from build123d import *

# Parameters (mm, degrees)
SKETCH1_W           = 44.45
SKETCH1_H           = 50.8
BOSS_EXTRUDE1_DEPTH = 76.2
CUT_EXTRUDE1_REACH  = 93.801
SKETCH2_R           = 6.731
SKETCH3_R           = 9.906
CUT_EXTRUDE2_DEPTH  = 38.608
CUT_EXTRUDE3_DEPTH  = 6.35


with BuildPart() as part:
    # Sketch1 → Boss-Extrude1 (new, symmetric)
    with BuildSketch(Plane.XY):
        Rectangle(SKETCH1_W, SKETCH1_H)
    extrude(amount=BOSS_EXTRUDE1_DEPTH, both=True)

    # Sketch2 → Cut-Extrude1 (cut, up to next)
    with BuildSketch(Plane(origin=(22.225, 0, 0), x_dir=(0, 0, -1), z_dir=(1, 0, 0)), mode=Mode.PRIVATE) as cut_extrude1_sk1:
        with Locations((-49.2125, -1.524)):
            Circle(SKETCH2_R)
    cut_extrude1_tool1 = extrude(cut_extrude1_sk1.sketch, amount=-CUT_EXTRUDE1_REACH, mode=Mode.PRIVATE) & part.part
    # Sketch2 → Cut-Extrude1 (cut, up to next)
    with BuildSketch(Plane(origin=(22.225, 0, 0), x_dir=(0, 0, -1), z_dir=(1, 0, 0)), mode=Mode.PRIVATE) as cut_extrude1_sk2:
        with Locations((49.2125, -1.524)):
            Circle(SKETCH2_R)
    cut_extrude1_tool2 = extrude(cut_extrude1_sk2.sketch, amount=-CUT_EXTRUDE1_REACH, mode=Mode.PRIVATE) & part.part
    add(cut_extrude1_tool1.solids().sort_by_distance((22.225, -1.524, 49.2125))[0], mode=Mode.SUBTRACT)
    add(cut_extrude1_tool2.solids().sort_by_distance((22.225, -1.524, -49.2125))[0], mode=Mode.SUBTRACT)

    # Sketch3 → Cut-Extrude2 (cut)
    with BuildSketch(Plane(origin=(22.225, 0, 0), x_dir=(0, 0, -1), z_dir=(1, 0, 0))):
        with Locations((-49.2125, -1.524)):
            Circle(SKETCH3_R)
        with Locations((49.2125, -1.524)):
            Circle(SKETCH3_R)
    extrude(amount=-CUT_EXTRUDE2_DEPTH, mode=Mode.SUBTRACT)

    # Sketch4 → Cut-Extrude3 (cut)
    with BuildSketch(Plane.XZ.offset(25.4)):
        with BuildLine():
            Line((22.225, -12.890241244), (22.225, 21.531765175))
            Line((22.225, 21.531765175), (0.947246364, 18.89010908))
            ThreePointArc((0.947246364, 18.89010908), (-11.925153457, 4.320761965), (0.947246364, -10.248585149))
            Line((0.947246364, -10.248585149), (22.225, -12.890241244))
        make_face()
    extrude(amount=-CUT_EXTRUDE3_DEPTH, mode=Mode.SUBTRACT)


solid = part.part
Can you work these out from the model? Positions are in its coordinate system, mm. A direction names the side the tool comes from. Coordinates: 2 decimals unless noted, no trailing zeros. Write each loop counter-clockwise with the first axis right and the second up, starting at its lowest first coordinate (ties: lowest second). Pieces come first, ordered by that corner, then holes.
Q1. Imagine slicing it at A-A, the plane y = -22. List the corners of the cut face in (x, z) for me (3 decimals).
Results found:
outline: (-22.225, -76.2) - (22.225, -76.2) - (22.225, -12.89) - (0.947, -10.249) arc R14.681 cw to (0.947, 18.89) - (22.225, 21.532) - (22.225, 76.2) - (-22.225, 76.2) - close
Q2. For P1, Ø10, axis at x = 8, z = 1, coming from the -Y side; P2, Ø6, axis at y = -0.5, z = 44.5, coming from the +X side; P3, Ø12, axis at x = 5.5, z = -5.5, coming from the -Y side, each with a flat end and sliding along its axis, tell me the tip position at first contact or that it passes through.
Results found:
P1: stops at y = -19.05
P2: stops at x = -16.38
P3: stops at y = -25.4
Q3. Which directions (+Z, -Z, +X, -X, +Y, -Y) give clear straight access to the entire face, cutting with the end or side of a thin tool? Please do faces 5 (the face through (-19.263, -4.102, 42.995)), 6 (the face through (-16.383, -4, -56)), 7 (the face through (-11.922, -22.269, 4.618)).
Results found:
face 5: +X, -X
face 6: +X
face 7: +X, -Y
Q4. Imagine slicing it at C-C, the plane z = 44.5. List the corners of the cut face in (x, y) for me (3 decimals).
Results found:
outline: (-22.225, -25.4) - (22.225, -25.4) - (22.225, -10.237) - (-16.383, -10.237) - (-16.383, -6.33) - (-22.225, -6.33) - close; (-22.225, 3.282) - (-16.383, 3.282) - (-16.383, 7.189) - (22.225, 7.189) - (22.225, 25.4) - (-22.225, 25.4) - close
Q5. If we mould it in two halves opening along Z, with no side actions, what happens to faces 1 (the face through (0, 0, 76.2)), 2 (the face through (11.74, -22.27, 20.23)), 3 (the face through (0, 0, -76.2)), 4 (the face through (0, 25.4, 1))? For each: +Z half, -Z half, draft (parallel to the pull), parting line (faces both ways), or undercut.
Results found:
face 1: +Z half
face 2: undercut
face 3: -Z half
face 4: draft
Q6. Imagine slicing it at D-D, the plane y = -5. List the corners of the cut face in (x, z) for me (1 decimal), plus the area to 3 significant figures.
Results found:
outline: (-22.2, -76.2) - (22.2, -76.2) - (22.2, -58.5) - (-16.4, -58.5) - (-16.4, -55) - (-22.2, -55) - close; (-22.2, -43.4) - (-16.4, -43.4) - (-16.4, -39.9) - (22.2, -39.9) - (22.2, 39.9) - (-16.4, 39.9) - (-16.4, 43.4) - (-22.2, 43.4) - close; (-22.2, 55) - (-16.4, 55) - (-16.4, 58.5) - (22.2, 58.5) - (22.2, 76.2) - (-22.2, 76.2) - close
area: 5,210 mm2
Q7. Please list where these lines run through material, in increasing order: L1, parallel to Z at x = 9, y = -7; L2, parallel to Z at x = -10, y = -6; L3, parallel to Y at x = -7, z = -45.5.
Results found:
L1: z = -76.2 to -57.47, -40.96 to 40.96, 57.47 to 76.2
L2: z = -76.2 to -58.05, -40.38 to 40.38, 58.05 to 76.2
L3: y = -25.4 to -10.71, 7.66 to 25.4
Q8. Imagine slicing it at B-B, the plane x = 3. List the corners of the cut face in (y, z) for me, plus the area to 3 significant figures.
Results found:
outline: (-25.4, -76.2) - (25.4, -76.2) - (25.4, 76.2) - (-25.4, 76.2) - (-25.4, 19.14) - (-19.05, 19.14) - (-19.05, -10.5) - (-25.4, -10.5) - close; hole circle Ø19.81 at (-1.52, -49.21); hole circle Ø19.81 at (-1.52, 49.21)
area: 6,940 mm2
